```python
from build123d import *

# Parameters (mm, degrees)
SKETCH1_W           = 160
SKETCH1_H           = 160
SKETCH1_R           = 1.5
BOSS_EXTRUDE1_DEPTH = 4
SKETCH5_W           = 160
SKETCH5_H           = 75
BOSS_EXTRUDE4_DEPTH = 4
FILLET1_R           = 3
FILLET2_R           = 3
FILLET3_R           = 3
CUT_EXTRUDE6_DEPTH  = 165
FILLET8_R           = 2
FILLET9_R           = 2
SKETCH13_W          = 100
SKETCH13_H          = 25
CUT_EXTRUDE7_DEPTH  = 10
SKETCH17_W          = 71.2
SKETCH17_H          = 24.5
CUT_EXTRUDE10_DEPTH = 10
SKETCH20_R          = 2.5
BOSS_EXTRUDE5_DEPTH = 3.2
SKETCH21_W          = 11.8
SKETCH21_H          = 21.1
CUT_EXTRUDE11_DEPTH = 5
SKETCH23_R          = 2.55
CUT_EXTRUDE12_DEPTH = 4
SKETCH24_R          = 4
BOSS_EXTRUDE6_DEPTH = 4
SKETCH25_R          = 2.55
CUT_EXTRUDE15_DEPTH = 4
SKETCH26_R          = 3.5
CUT_EXTRUDE16_DEPTH = 10


with BuildPart() as part:
    # Sketch1 → Boss-Extrude1 (new body)
    with BuildSketch(Plane(origin=(0, 0, 0), x_dir=(1, 0, 0), z_dir=(0, 1, 0))):
        Rectangle(SKETCH1_W, SKETCH1_H)
        with Locations(Location((-73.75, 73.75, 0), (0, 0, 270))):
            Circle(SKETCH1_R, mode=Mode.SUBTRACT)
        with Locations(Location((73.75, 73.75, 0), (0, 0, 270))):
            Circle(SKETCH1_R, mode=Mode.SUBTRACT)
        with Locations(Location((-73.75, -77.75, 0), (0, 0, 270))):
            Circle(SKETCH1_R, mode=Mode.SUBTRACT)
        with Locations(Location((73.75, -77.75, 0), (0, 0, 270))):
            Circle(SKETCH1_R, mode=Mode.SUBTRACT)
    extrude(amount=BOSS_EXTRUDE1_DEPTH)

    # Sketch5 → Boss-Extrude4 (add)
    with BuildSketch(Plane(origin=(0, 34.641016151, 20), x_dir=(1, 0, 0), z_dir=(0, 0.8660254037844346, 0.5000000000000071))):
        with Locations((0, -104.782032303)):
            Rectangle(SKETCH5_W, SKETCH5_H)
    extrude(amount=BOSS_EXTRUDE4_DEPTH)

    # Fillet1
    # the kernel refuses this fillet: 3 mm, written as the material it takes off along each edge
    with BuildSketch(Plane(origin=(-84.277998386, 4.464101615, 80.267949192), x_dir=(0, -0.8660254037849107, -0.4999999999991824), z_dir=(1, 0, 0))) as fillet1_piece_1:
        with BuildLine():
            CenterArc((3, -1.711199354), FILLET1_R, 145.221891332, 34.778108668)
            Line((0, -1.711199354), (-0.06, -1.711199354))
            Line((-0.06, -1.711199354), (-0.06, 0))
            Line((-0.06, 0), (0, 0.06))
            ThreePointArc((0, 0.06), (0.267949192, 0.06), (0.486616353, 0.034223987))
            Line((0.486616353, 0.034223987), (0.535898385, 0))
        make_face()
    extrude(amount=168.555996772, mode=Mode.SUBTRACT)

    # Fillet2
    fillet2_edges = [part.edges().sort_by_distance(p)[0] for p in [
        (80, 2, -80),
    ]]
    fillet(fillet2_edges, radius=FILLET2_R)

    # Fillet3
    fillet3_edges = [part.edges().sort_by_distance(p)[0] for p in [
        (-80, 2, -80),
    ]]
    fillet(fillet3_edges, radius=FILLET3_R)

    # Sketch12 → Cut-Extrude6 (cut)
    with BuildSketch(Plane(origin=(80, 0, 0), x_dir=(0, 0, -1), z_dir=(1, 0, 0))):
        Polygon((-145.219854476, -33.035898385), (-143.219854476, -36.5), (-141.002829443, -35.22), (-141.002829443, -30.601197846), align=None)
    extrude(amount=-CUT_EXTRUDE6_DEPTH, mode=Mode.SUBTRACT)

    # Fillet8
    fillet8_edges = [part.edges().sort_by_distance(p)[0] for p in [
        (80, -32.910598923, 141.002829443),
    ]]
    fillet(fillet8_edges, radius=FILLET8_R)

    # Fillet9
    fillet9_edges = [part.edges().sort_by_distance(p)[0] for p in [
        (-80, -32.910598923, 141.002829443),
    ]]
    fillet(fillet9_edges, radius=FILLET9_R)

    # Sketch13 → Cut-Extrude7 (cut)
    with BuildSketch(Plane(origin=(0, 4, 0), x_dir=(1, 0, 0), z_dir=(0, 1, 0))):
        with Locations((5, 0)):
            Rectangle(SKETCH13_W, SKETCH13_H)
    extrude(amount=-CUT_EXTRUDE7_DEPTH, mode=Mode.SUBTRACT)

    # Sketch17 → Cut-Extrude10 (cut)
    with BuildSketch(Plane(origin=(0, 38.105117767, 22), x_dir=(1, 0, 0), z_dir=(0, 0.8660254037844344, 0.5000000000000073))):
        with Locations((0, -103.993231657)):
            Rectangle(SKETCH17_W, SKETCH17_H)
    extrude(amount=-CUT_EXTRUDE10_DEPTH, mode=Mode.SUBTRACT)

    # Sketch20 → Boss-Extrude5 (add)
    with BuildSketch(Plane(origin=(0, 34.641016151, 20), x_dir=(1, 0, 0), z_dir=(0, -0.8660254037844344, -0.5000000000000073))):
        with Locations(Location((-37.592365001, 119.501924995, 0), (0, 0, 270))):
            Circle(SKETCH20_R)
        with Locations(Location((37.567634999, 88.501924995, 0), (0, 0, 270))):
            Circle(SKETCH20_R)
        with Locations(Location((37.567634999, 119.501924995, 0), (0, 0, 270))):
            Circle(SKETCH20_R)
        with Locations(Location((-37.592365001, 88.501924995, 0), (0, 0, 270))):
            Circle(SKETCH20_R)
    extrude(amount=BOSS_EXTRUDE5_DEPTH)

    # Sketch21 → Cut-Extrude11 (cut)
    with BuildSketch(Plane(origin=(0, 38.105117767, 22), x_dir=(1, 0, 0), z_dir=(0, 0.8660254037844344, 0.5000000000000073))):
        with Locations((57.997068985, -110.479162625)):
            Rectangle(SKETCH21_W, SKETCH21_H)
    extrude(amount=-CUT_EXTRUDE11_DEPTH, mode=Mode.SUBTRACT)

    # Sketch23 → Cut-Extrude12 (cut)
    with BuildSketch(Plane(origin=(0, 38.105117767, 22), x_dir=(1, 0, 0), z_dir=(0, 0.8660254037844345, 0.5000000000000074))):
        with Locations(Location((58.097068985, -91.429162625, 0), (0, 0, 270))):
            Circle(SKETCH23_R)
    extrude(amount=-CUT_EXTRUDE12_DEPTH, mode=Mode.SUBTRACT)

    # Sketch24 → Boss-Extrude6 (add)
    with BuildSketch(Plane(origin=(0, 34.641016151, 20), x_dir=(1, 0, 0), z_dir=(0, -0.8660254037844344, -0.5000000000000073))):
        with Locations(Location((58.097068985, 91.429162625, 0), (0, 0, 90))):
            Circle(SKETCH24_R)
    extrude(amount=BOSS_EXTRUDE6_DEPTH)

    # Sketch25 → Cut-Extrude15 (cut)
    with BuildSketch(Plane(origin=(0, 34.641016151, 20), x_dir=(1, 0, 0), z_dir=(0, -0.8660254037844345, -0.5000000000000074))):
        with Locations(Location((58.097068985, 91.429162625, 0), (0, 0, 90))):
            Circle(SKETCH25_R)
    extrude(amount=CUT_EXTRUDE15_DEPTH, mode=Mode.SUBTRACT)

    # Sketch26 → Cut-Extrude16 (cut)
    with BuildSketch(Plane(origin=(0, 38.105117767, 22), x_dir=(1, 0, 0), z_dir=(0, 0.8660254037844345, 0.5000000000000074))):
        with Locations(Location((-59.8, -98.912631226, 0), (0, 0, 270))):
            Circle(SKETCH26_R)
    extrude(amount=-CUT_EXTRUDE16_DEPTH, mode=Mode.SUBTRACT)


solid = part.part
```
Geometry check sheet. Reference: the model listing, model coordinates, mm. A direction names the side the tool comes from. Give positions to 0.01 mm unless a question says otherwise; leave off trailing zeros. Order: outer loops, then holes, each group sorted by start corner. A loop starts at its lowest first (then second) coordinate and runs counter-clockwise, first axis right, second up. Notation, with made-up numbers: (-21.75, 22) - (22.25, 22) arc R28 cw to (22.25, 48) - close; hole circle Ø1 at (61, 20.5). An arc over 180 degrees is marked (long way). Answer in a Markdown table with one row per item. Add a question column.
Q1. Gauge pin test, flat ends, axial feed: pin 1 (3 mm diameter, centred on x = 0.5, y = 2, fed in from +Z); pin 2 (3 mm diameter, centred on x = 21, y = -3, fed in from +Z); pin 3 (3 mm diameter, centred on x = 11, z = 67.5, fed in from +Y). Record the tip position at first contact, or that the pin passes through.
Q2. Tool access check on faces 5 (the flat face through (-37.56, -12.4, 95.08)), 6 (the flat face through (-1.12, -5.65, 97.79)). Record the directions out of +Z, -Z, +X, -X, +Y, -Y that give a thin tool (end or side, any length) a straight path to the whole face; none if there is none.
Q3. Mould release check, pull along Z, two halves, no side actions. Record for faces 1 (the flat face through (63.897, -19, 117)), 2 (the flat face through (1, -33, 141.003)), 3 (the cylindrical face through (39.26, -11.9, 97.45)), 4 (the cylindrical face through (-63.217, -12.68, 106.018)): pulls with the +Z half, pulls with the -Z half, needs draft (parallel to the pull), parting line crosses it, or undercut.
Q4. Material ranges on probe 1 along X at (y, z) = (1.4, 77.75); probe 2 along Z at (x, y) = (-73, 2); probe 3 along Z at (x, y) = (73, 1), recorded low to high. Write a range as from..to.
Q5. Cross-section at B-B, the plane z = -23. Enter the section's corners in (x, y).
Q6. Cross-section at A-A, the plane x = 10. Enter the section's corners in (y, z).
Check values:
| question | item | result |
|---|---|---|
| 1 | pin 1 | stops at z = 87.13 |
| 1 | pin 2 | stops at z = 95.79 |
| 1 | pin 3 | stops at y = 4 |
| 2 | face 5 | -Z, -X, -Y |
| 2 | face 6 | +Z, +X, -X, +Y |
| 3 | face 1 | needs draft |
| 3 | face 2 | pulls with the +Z half |
| 3 | face 3 | undercut |
| 3 | face 4 | undercut |
| 4 | probe 1 | x = -80..-75.25, -72.25..72.25, 75.25..80 |
| 4 | probe 2 | z = -80..-75.05, -72.45..76.45, 78.85..84.54 |
| 4 | probe 3 | z = -80..-75.05, -72.45..76.45, 78.27..86.27 |
| 5 | outline | (-80, 0) - (80, 0) - (80, 4) - (-80, 4) - close |
| 6 | outline | (-35.22, 141) - (-23.48, 120.67) - (-20.02, 122.67) - (-30.6, 141) - close; (-11.23, 99.45) - (0, 80) - (0, 12.5) - (4, 12.5) - (4, 80) arc R3 ccw to (3.61, 81.75) - (-7.77, 101.45) - close; (0, -80) - (4, -80) - (4, -12.5) - (0, -12.5) - close |
